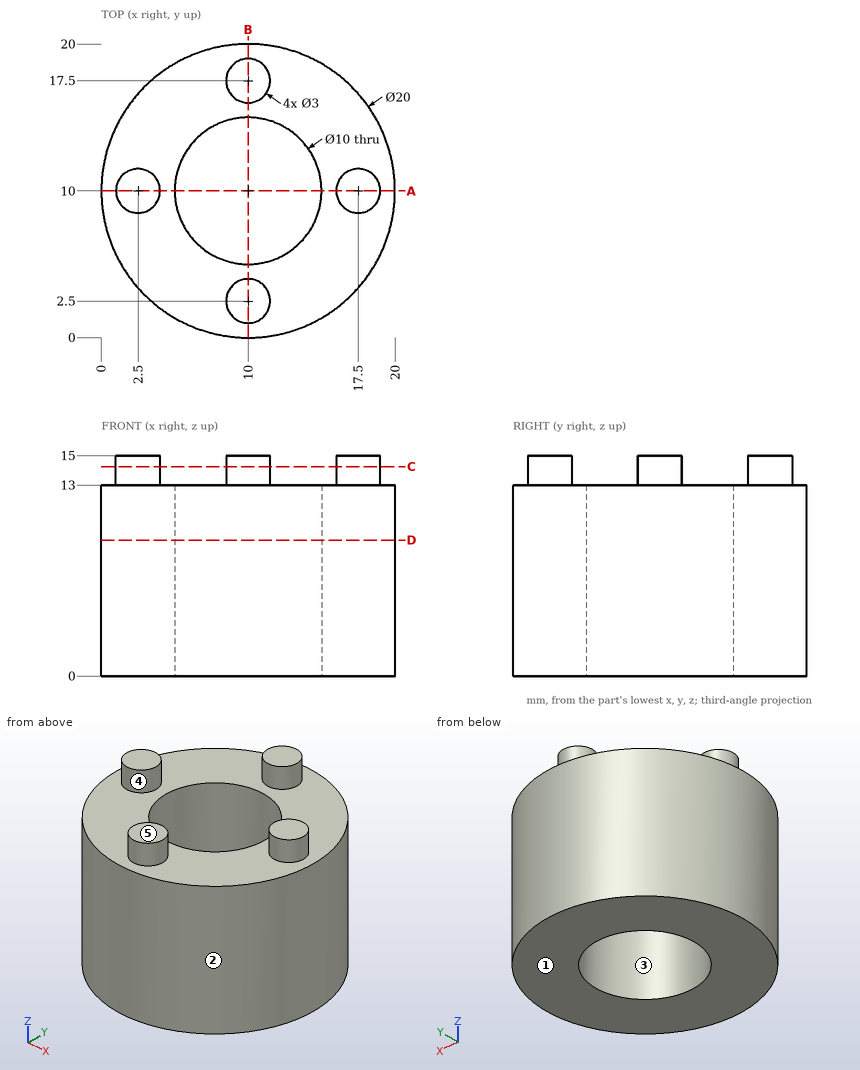
Source: three-view drawing plus pictorial views. Frame: mm from the lowest corner of the part. A direction names the side the tool comes from. Round coordinates to 2 decimals unless told otherwise and drop trailing zeros. Order: outer loops, then holes, each group sorted by start corner. A loop starts at its lowest first (then second) coordinate and runs counter-clockwise, first axis right, second up. Notation, with made-up numbers: (9.5, 7) - (37.5, 7) arc R24 ccw to (37.5, 18) - close; hole circle Ø1 at (1.5, 29). An arc over 180 degrees is marked (long way). Write each question's results on one line, items separated by ' | '.
Item 1: Section A-A, the plane y = 10. Return the cut outline in (x, z), and give its area (3 significant figures).
Completed:
outline: (0, 0) - (5, 0) - (5, 13) - (4, 13) - (4, 15) - (1, 15) - (1, 13) - (0, 13) - close; (15, 0) - (20, 0) - (20, 13) - (19, 13) - (19, 15) - (16, 15) - (16, 13) - (15, 13) - close | area: 142 mm^2
Item 2: Section C-C, the plane z = 14.25. Return the cut outline in (x, y).
Completed:
outline: circle Ø3 at (2.5, 10); circle Ø3 at (10, 2.5); circle Ø3 at (10, 17.5); circle Ø3 at (17.5, 10)
Item 3: Mould query, pull axis X, two halves, no side actions, for the marked faces 1, 2 and 3. Classes: pulls with the +X half, pulls with the -X half, needs draft (parallel to the pull), parting line crosses it, or undercut.
Completed:
face 1: needs draft | face 2: parting line crosses it | face 3: undercut
Item 4: Reachability of the marked faces 4 and 5 from +Z, -Z, +X, -X, +Y, -Y: full face, straight path, thin tool, end or side. Return the list, or none.
Completed:
face 4: +Z | face 5: +Z, +X, -X, +Y, -Y
Item 5: Section D-D, the plane z = 9.25. Return the cut outline in (x, y), and give its area (3 significant figures).
Completed:
outline: circle Ø20 at (10, 10); hole circle Ø10 at (10, 10) | area: 236 mm^2
Item 6: First-contact query: pin 1 Ø1 at (y, z) = (4, 13) entering from -X; pin 2 Ø1.5 at (y, z) = (12.5, 12) entering from +X; pin 3 Ø3 at (x, z) = (9.5, 2.5) entering from -Y; pin 4 Ø4 at (y, z) = (13, 2) entering from -X. Flat tips, straight axial feed; report the tip coordinate or a pass-through.
Completed:
pin 1: x = 1.65 | pin 2: x = 19.85 | pin 3: y = 0 | pin 4: x = 0.05
Item 7: Material intervals for line 1 along Y through (x, z) = (10, 10); line 2 along Z through (x, y) = (16.5, 16); line 3 along X through (y, z) = (2, 8.5), sorted ascending. Write a range as [from, to].
Completed:
line 1: [0, 5], [15, 20] | line 2: [0, 13] | line 3: [4, 16]
